Geometry: final body of the model. Coordinates: model frame, mm. A direction names the side the tool comes from. Round coordinates to 2 decimals unless told otherwise and drop trailing zeros. Loops run counter-clockwise (first coordinate to the right, second up) from the corner with the lowest first, then second, coordinate; pieces in that order, holes last. Notation, with made-up numbers: (-2, -16.75) - (29, -16.75) arc R18 cw to (29, 7.25) - close; hole circle Ø2 at (-0.5, 21.25). An arc over 180 degrees is marked (long way). Answer as CSV lines item,"result".
from build123d import *

# Parameters (mm, degrees)
SKETCH1_R                = 22.5
SKETCH1_R_2              = 16.9
BOSS_EXTRUDE1_DEPTH      = 19
BOSS_EXTRUDE2_DEPTH      = 11
BOSS_EXTRUDE2_DEPTH_BACK = 7
BOSS_EXTRUDE3_DEPTH      = 15
BOSS_EXTRUDE3_DEPTH_BACK = 11
BOSS_EXTRUDE4_DEPTH      = 9
FILLET1_RADIUS           = 9
FILLET1_LENGTH           = 30
FILLET2_RADIUS           = 9
FILLET2_LENGTH           = 30
SKETCH2_R                = 4.5
CUT_EXTRUDE1_DEPTH       = 78
FILLET5_R                = 22.5
BOSS_EXTRUDE5_DEPTH      = 5


with BuildPart() as part:
    # Sketch1 → Boss-Extrude1 (new, symmetric)
    with BuildSketch(Plane.XY):
        with Locations((0, 201.2)):
            Circle(SKETCH1_R)
        with Locations((0, 201.2)):
            Circle(SKETCH1_R_2, mode=Mode.SUBTRACT)
    extrude(amount=BOSS_EXTRUDE1_DEPTH, both=True)

    # Sketch1<3> → Boss-Extrude2 (add, two sides: drawn at the far end of the back side and taken through both)
    with BuildSketch(Plane.XY.offset(-BOSS_EXTRUDE2_DEPTH_BACK)):
        with BuildLine():
            ThreePointArc((-22.483530605, 30), (-24.572828472, 26.825646402), (-26.953938029, 23.863889556))
            ThreePointArc((-26.953938029, 23.863889556), (0, 36), (26.953938029, 23.863889556))
            ThreePointArc((26.953938029, 23.863889556), (24.572828472, 26.825646402), (22.483530605, 30))
            ThreePointArc((22.483530605, 30), (18.612945898, 38.808225452), (16.957576671, 48.285884145))
            Line((16.957576671, 48.285884145), (10, 181.044355629))
            ThreePointArc((10, 181.044355629), (0, 178.7), (-10, 181.044355629))
            Line((-10, 181.044355629), (-16.957576671, 48.285884145))
            ThreePointArc((-16.957576671, 48.285884145), (-18.612945898, 38.808225452), (-22.483530605, 30))
        make_face()
        with BuildLine():
            ThreePointArc((-8, 145), (0, 153), (8, 145))
            Line((8, 145), (8, 55))
            ThreePointArc((8, 55), (0, 47), (-8, 55))
            Line((-8, 55), (-8, 145))
        make_face(mode=Mode.SUBTRACT)
    extrude(amount=BOSS_EXTRUDE2_DEPTH + BOSS_EXTRUDE2_DEPTH_BACK)

    # Sketch1<4> → Boss-Extrude3 (add, two sides: drawn at the far end of the back side and taken through both)
    with BuildSketch(Plane.XY.offset(-BOSS_EXTRUDE3_DEPTH_BACK)):
        with BuildLine():
            ThreePointArc((-26.953938029, 23.863889556), (-33.66260365, 12.760451225), (-36, 0))
            Line((-36, 0), (-27, 0))
            ThreePointArc((-27, 0), (0, 27), (27, 0))
            Line((27, 0), (36, 0))
            ThreePointArc((36, 0), (33.66260365, 12.760451225), (26.953938029, 23.863889556))
            ThreePointArc((26.953938029, 23.863889556), (0, 36), (-26.953938029, 23.863889556))
        make_face()
    extrude(amount=BOSS_EXTRUDE3_DEPTH + BOSS_EXTRUDE3_DEPTH_BACK)

    # Sketch1<6> → Boss-Extrude4 (add, symmetric)
    with BuildSketch(Plane.XY):
        with BuildLine():
            Line((-47, 0), (-36, 0))
            ThreePointArc((-36, 0), (-33.66260365, 12.760451225), (-26.953938029, 23.863889556))
            ThreePointArc((-26.953938029, 23.863889556), (-24.572828472, 26.825646402), (-22.483530605, 30))
            Line((-22.483530605, 30), (-47, 30))
            Line((-47, 30), (-47, 0))
        make_face()
        with BuildLine():
            ThreePointArc((22.483530605, 30), (24.572828472, 26.825646402), (26.953938029, 23.863889556))
            ThreePointArc((26.953938029, 23.863889556), (33.66260365, 12.760451225), (36, 0))
            Line((36, 0), (47, 0))
            Line((47, 0), (47, 30))
            Line((47, 30), (22.483530605, 30))
        make_face()
    extrude(amount=BOSS_EXTRUDE4_DEPTH, both=True)

    # Fillet1: full round fillet: the end face becomes a half cylinder, R = half its width
    fillet1_face = Plane((47, 15, 0), x_dir=(0, 1, 0), z_dir=(1, 0, 0))  # on the end face: x along it, z out of the body
    fillet1_slab = fillet1_face.offset(-FILLET1_RADIUS / 2) * Box(FILLET1_LENGTH, 2 * FILLET1_RADIUS, FILLET1_RADIUS, mode=Mode.PRIVATE)  # the body's end, R deep
    fillet1_round = Plane((38, 15, 0), x_dir=(1, 0, 0), z_dir=(0, 1, 0)) * Cylinder(FILLET1_RADIUS, FILLET1_LENGTH, mode=Mode.PRIVATE)  # its axis R under the face
    add(fillet1_slab - fillet1_round, mode=Mode.SUBTRACT)

    # Fillet2: full round fillet: the end face becomes a half cylinder, R = half its width
    fillet2_face = Plane((-47, 15, 0), x_dir=(0, 1, 0), z_dir=(-1, 0, 0))  # on the end face: x along it, z out of the body
    fillet2_slab = fillet2_face.offset(-FILLET2_RADIUS / 2) * Box(FILLET2_LENGTH, 2 * FILLET2_RADIUS, FILLET2_RADIUS, mode=Mode.PRIVATE)  # the body's end, R deep
    fillet2_round = Plane((-38, 15, 0), x_dir=(-1, 0, 0), z_dir=(0, 1, 0)) * Cylinder(FILLET2_RADIUS, FILLET2_LENGTH, mode=Mode.PRIVATE)  # its axis R under the face
    add(fillet2_slab - fillet2_round, mode=Mode.SUBTRACT)

    # Sketch2 → Cut-Extrude1 (cut)
    with BuildSketch(Plane(origin=(0, 30, 0), x_dir=(1, 0, 0), z_dir=(0, 1, 0))):
        with Locations(Location((38, 0, 0), (0, 0, 270))):
            Circle(SKETCH2_R)
        with Locations(Location((-38, 0, 0), (0, 0, 270))):
            Circle(SKETCH2_R)
    extrude(amount=-CUT_EXTRUDE1_DEPTH, mode=Mode.SUBTRACT)

    # Fillet5
    fillet5_edges = [part.edges().sort_by_distance(p)[0] for p in [
        (-10, 181.044355629, 2),
        (10, 181.044355629, 2),
    ]]
    fillet(fillet5_edges, radius=FILLET5_R)

    # Sketch1<7> → Boss-Extrude5 (add, symmetric)
    with BuildSketch(Plane.XY):
        with BuildLine():
            Line((-8, 145), (-8, 55))
            ThreePointArc((-8, 55), (0, 47), (8, 55))
            Line((8, 55), (8, 145))
            ThreePointArc((8, 145), (0, 153), (-8, 145))
        make_face()
    extrude(amount=BOSS_EXTRUDE5_DEPTH, both=True)


solid = part.part
(1) Material intervals for line 1 along Y through (x, z) = (0, 7); line 2 along Y through (x, z) = (0, 1); line 3 along X through (y, z) = (13, -0.5), sorted ascending.
Findings below:
line 1,"27 to 47, 153 to 184.3, 218.1 to 223.7"
line 2,"27 to 184.3, 218.1 to 223.7"
line 3,"-46.99 to -42.47, -33.53 to -23.66, 23.66 to 33.53, 42.47 to 46.99"
(2) Draft query along X for faces 1 (the face through (-34, 22, -9)), 2 (the face through (-13.737, 109.746, 1.874)), 3 (the face through (0, 153, 8)). Return one class per face: pulls with the +X half, pulls with the -X half, needs draft (parallel to the pull), parting line crosses it, or undercut.
Findings below:
face 1,"needs draft"
face 2,"pulls with the -X half"
face 3,"undercut"
(3) Pin query (flat end, axial travel): P1, Ø5, axis at y = 97, z = 3, coming from the +X side; P2, Ø2, axis at y = 98.5, z = -6, coming from the -X side; P3, Ø14.5, axis at x = -36, z = -4, coming from the +Y side; P4, Ø14.5, axis at x = 38, z = 0, coming from the -Y side. Return the tip coordinate at first contact, or that it passes through.
Findings below:
P1,"x = 14.54"
P2,"x = -14.38"
P3,"y = 30"
P4,"y = 0"
(4) Section B-B (y = 201.2). Output: boundary loops of the cut face in (x, z).
Findings below:
outline,"(-22.5, -19) - (-16.9, -19) - (-16.9, 19) - (-22.5, 19) - close; (16.9, -19) - (22.5, -19) - (22.5, 19) - (16.9, 19) - close"
(5) Section D-D (y = 102.5). Output: boundary loops of the cut face in (x, z).
Findings below:
outline,"(-14.12, -7) - (-8, -7) - (-8, -5) - (8, -5) - (8, -7) - (14.12, -7) - (14.12, 11) - (8, 11) - (8, 5) - (-8, 5) - (-8, 11) - (-14.12, 11) - close"
(6) Section A-A (z = 0). Output: boundary loops of the cut face in (x, y).
Findings below:
outline,"(-47, 0) - (-42.5, 0) - (-42.5, 30) - (-47, 30) - close; (-33.5, 0) - (-27, 0) arc R27 cw to (27, 0) - (33.5, 0) - (33.5, 30) - (22.48, 30) arc R40 cw to (16.96, 48.29) - (10.6, 169.51) arc R22.5 cw to (16.54, 185.94) arc R22.5 ccw (long way) to (-16.54, 185.94) arc R22.5 cw to (-10.6, 169.51) - (-16.96, 48.29) arc R40 cw to (-22.48, 30) - (-33.5, 30) - close; (42.5, 0) - (47, 0) - (47, 30) - (42.5, 30) - close; hole circle Ø33.8 at (0, 201.2)"
(7) Section C-C (x = 2). Output: boundary loops of the cut face in (y, z), and give its area (3 significant figures).
Findings below:
outline,"(26.93, -11) - (35.94, -11) - (35.94, -7) - (47.25, -7) - (47.25, -5) - (152.75, -5) - (152.75, -7) - (178.79, -7) - (178.79, -19) - (184.42, -19) - (184.42, 19) - (178.79, 19) - (178.79, 11) - (152.75, 11) - (152.75, 5) - (47.25, 5) - (47.25, 11) - (35.94, 11) - (35.94, 15) - (26.93, 15) - close; (217.98, -19) - (223.61, -19) - (223.61, 19) - (217.98, 19) - close"
area,"2,390 mm2"
(8) Access query for faces 4 (the face through (-1, 30, 15)), 5 (the face through (32, 30, 0)), 6 (the face through (0, 153, -6)), 7 (the face through (-32, 30, 0)), 8 (the face through (13.826, 108.048, 1.874)). Directions: +Z, -Z, +X, -X, +Y, -Y. A direction counts if a zero-diameter tool reaches every point of the face in a straight line with its end or side. Return the directions, or none.
Findings below:
face 4,"+Z, +X, -X, -Y"
face 5,"+Z, -Z, +X, +Y"
face 6,"-Z"
face 7,"+Z, -Z, -X, +Y"
face 8,"+Z, -Z, +X"
